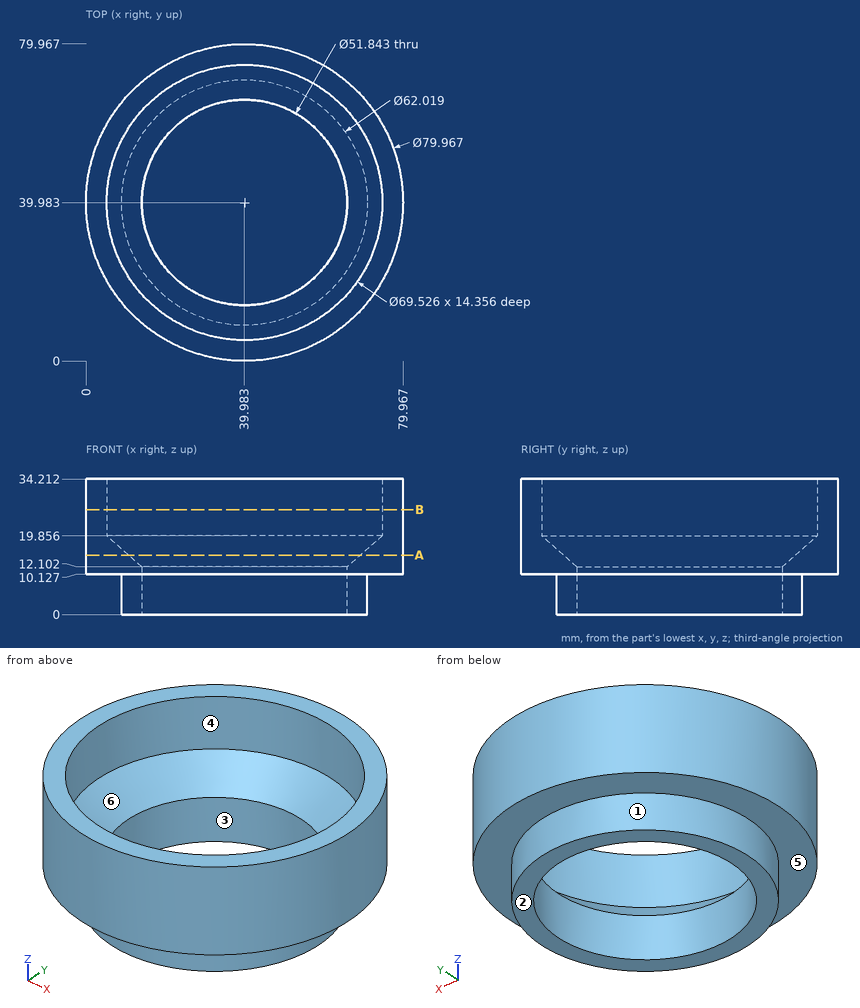
Here's the drawing with two shaded views (mm, measured from the low corner). I have some questions. A direction names the side the tool comes from. Coordinates: 2 decimals unless noted, no trailing zeros. Write each loop counter-clockwise with the first axis right and the second up, starting at its lowest first coordinate (ties: lowest second). Pieces come first, ordered by that corner, then holes. Notation, with made-up numbers: (-15, -31) -> (24, -31) arc R31 cw to (24, -1) -> close; hole circle Ø9 at (78.5, 77.25). An arc over 180 degrees is marked (long way). Use a Markdown table: item, result. Add a question column.
(1) Please list where these lines run through material, in increasing order: line 1 (X direction, y = 41, z = 8) (1 decimal); line 2 (Y direction, x = 13, z = 28.5) (1 decimal); line 3 (X direction, y = 14.5, z = 29) (1 decimal).
(2) If we section it at A-A, the plane z = 15: Write out the boundary of the cut face in (x, y).
(3) For the marked faces 5 and 6, which set-ups out of +Z, -Z, +X, -X, +Y, -Y let a thin tool reach every point of the face, with its end or its side?
(4) We'd pull the mould along Y, two halves only. Please class the marked faces 1, 2, 3 and 4: +Y half, -Y half, draft (parallel to the pull), parting line (faces both ways), or undercut.
(5) If we section it at B-B, the plane z = 26.5: Write out the boundary of the cut face in (x, y) (1 decimal), and give its area (3 significant figures).
(6) I'm going to push flat-ended pins straight in: P1, Ø4, axis at x = 33, z = 24, coming from the +Y side (1 decimal); P2, Ø4, axis at y = 30.5, z = 14, coming from the -X side; P3, Ø4, axis at x = 53.5, z = 12.5, coming from the -Y side (1 decimal); P4, Ø12, axis at x = 41, y = 58.5, coming from the -Z side. Where does each tip first touch, or does it pass through?
Outcome:
| question | item | result |
|---|---|---|
| 1 | line 1 | x = 9 to 14.1, 65.9 to 71 |
| 1 | line 2 | y = 10.5 to 18.1, 61.9 to 69.5 |
| 1 | line 3 | x = 9.2 to 16.3, 63.6 to 70.8 |
| 2 | outline | circle Ø79.97 at (39.98, 39.98); hole circle Ø58.45 at (39.98, 39.98) |
| 3 | face 5 | -Z |
| 3 | face 6 | +Z |
| 4 | face 1 | parting line |
| 4 | face 2 | draft |
| 4 | face 3 | undercut |
| 4 | face 4 | undercut |
| 5 | outline | circle Ø80 at (40, 40); hole circle Ø69.5 at (40, 40) |
| 5 | area | 1,230 mm^2 |
| 6 | P1 | stops at y = 79.7 |
| 6 | P2 | stops at x = 0.71 |
| 6 | P3 | stops at y = 1.7 |
| 6 | P4 | passes through |
